Read the model definition and answer for the solid it produces. Units are mm, in the model's axes. Face numbers are marked on the shaded views. A direction names the side the tool comes from. Give positions to 0.01 mm unless a question says otherwise; leave off trailing zeros. Order: outer loops, then holes, each group sorted by start corner. A loop starts at its lowest first (then second) coordinate and runs counter-clockwise, first axis right, second up. Notation, with made-up numbers: (88, 43) -> (128, 43) arc R13 ccw to (128, 64) -> close; hole circle Ø3 at (9, 1). An arc over 180 degrees is marked (long way). One line per item, written item: value. Start each with the question number.
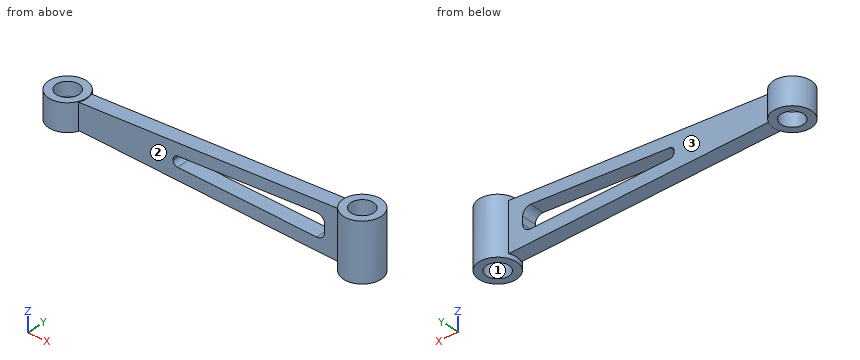
from build123d import *

# Parameters (mm, degrees)
SKETCH1_R           = 7.5
BOSS_EXTRUDE1_DEPTH = 9
SKETCH2_R           = 7.5
BOSS_EXTRUDE2_DEPTH = 19
BOSS_EXTRUDE3_DEPTH = 5
SKETCH4_R           = 12.5
BOSS_EXTRUDE4_DEPTH = 9
SKETCH6_R           = 12.5
BOSS_EXTRUDE5_DEPTH = 19
SKETCH7_R           = 7.5
CUT_EXTRUDE1_DEPTH  = 19
CUT_EXTRUDE2_DEPTH  = 19


with BuildPart() as part:
    # Sketch1 → Boss-Extrude1 (new body, symmetric)
    with BuildSketch(Plane.XY):
        Circle(SKETCH1_R)
    extrude(amount=BOSS_EXTRUDE1_DEPTH, both=True)



with BuildPart() as body_2:
    # Sketch2 → Boss-Extrude2 (new body, symmetric)
    with BuildSketch(Plane.XY):
        with Locations((194.56, 0)):
            Circle(SKETCH2_R)
    extrude(amount=BOSS_EXTRUDE2_DEPTH, both=True)


with BuildPart() as body_3:
    # Sketch3 → Boss-Extrude3 (new body, symmetric)
    with BuildSketch(Plane(origin=(0, 0, 0), x_dir=(1, 0, 0), z_dir=(0, 1, 0))):
        Polygon((7.5, 8.362970839), (187.06, 16.2), (187.06, -16.20477539), (7.5, -8.362286729), align=None)
    extrude(amount=BOSS_EXTRUDE3_DEPTH, both=True)


with BuildPart() as part_1:
    add(part.part)

    add(body_3.part)  # Boss-Extrude4 merges body 3
    # Sketch4 → Boss-Extrude4 (add, symmetric)
    with BuildSketch(Plane.XY):
        Circle(SKETCH4_R)
    extrude(amount=BOSS_EXTRUDE4_DEPTH, both=True)


    add(body_2.part)  # Boss-Extrude5 merges body 2
    # Sketch6 → Boss-Extrude5 (add, symmetric)
    with BuildSketch(Plane.XY):
        with Locations((194.56, 0)):
            Circle(SKETCH6_R)
    extrude(amount=BOSS_EXTRUDE5_DEPTH, both=True)

    # Sketch7 → Cut-Extrude1 (cut, symmetric)
    with BuildSketch(Plane.XY):
        Circle(SKETCH7_R)
        with Locations((194.56, 0)):
            Circle(SKETCH7_R)
    extrude(amount=CUT_EXTRUDE1_DEPTH, both=True, mode=Mode.SUBTRACT)

    # Sketch8 → Cut-Extrude2 (cut, symmetric)
    with BuildSketch(Plane(origin=(0, 5, 0), x_dir=(1, 0, 0), z_dir=(0, 1, 0))):
        with BuildLine():
            Line((76.769384169, 3.36885549), (168.688973616, 7.067498603))
            ThreePointArc((168.688973616, 7.067498603), (172.353731231, 5.677448491), (173.89, 2.071541398))
            Line((173.89, 2.071541398), (173.89, -2.721863896))
            ThreePointArc((173.89, -2.721863896), (172.341389234, -6.33958588), (168.654835057, -7.716330579))
            Line((168.654835057, -7.716330579), (76.748901034, -3.388930862))
            ThreePointArc((76.748901034, -3.388930862), (74.719366809, -2.463084392), (73.89, -0.392250852))
            Line((73.89, -0.392250852), (73.89, 0.371281167))
            ThreePointArc((73.89, 0.371281167), (74.726455744, 2.449519905), (76.769384169, 3.36885549))
        make_face()
    extrude(amount=CUT_EXTRUDE2_DEPTH, both=True, mode=Mode.SUBTRACT)


solid = part_1.part
Item 1: Find section B-B on y = 0. Write down the section's boundary in (x, z), then the cut area to 3 significant figures.
Item 2: Flat-ended cylindrical pins translate along their axes: pin 1 (6 mm diameter, centred on x = 175, y = -4, fed in from +Z); pin 2 (4 mm diameter, centred on x = 163.5, y = 1.5, fed in from +Z); pin 3 (9 mm diameter, centred on x = 194.56, y = 0, fed in from +Z); pin 4 (8 mm diameter, centred on y = -5, z = -7.5, fed in from +X). Find the tip coordinate at first contact, or state that the pin passes through.
Item 3: Find the intervals of material crossed by line 1 (Y direction, x = 194.56, z = -4); line 2 (X direction, y = 3.5, z = 8); line 3 (X direction, y = 10, z = -3), in increasing order. Write a range as from..to.
Item 4: Find section D-D on x = 194.56. Write down the section's boundary in (y, z), then the cut area to 3 significant figures.
Item 5: A tool of negligible diameter and unlimited length cuts with its end or side. For the marked faces 1, 2 and 3, from which of +Z, -Z, +X, -X, +Y, -Y can it reach the whole face along a straight path? Write none if from no direction.
Item 6: Find section A-A on x = 0. Write down the section's boundary in (y, z), then the cut area to 3 significant figures.
Item 7: Find section C-C on z = 12. Write down the section's boundary in (x, y).
Checks:
1. outline: (-12.5, -9) -> (-7.5, -9) -> (-7.5, 9) -> (-12.5, 9) -> close; (7.5, -9) -> (12.5, -9) -> (12.5, -8.58) -> (182.06, -15.98) -> (182.06, -19) -> (187.06, -19) -> (187.06, 19) -> (182.06, 19) -> (182.06, 15.99) -> (12.5, 8.58) -> (12.5, 9) -> (7.5, 9) -> close; (202.06, -19) -> (207.06, -19) -> (207.06, 19) -> (202.06, 19) -> close; hole (73.89, -0.37) arc R3 ccw to (76.77, -3.37) -> (168.69, -7.07) arc R5 ccw to (173.89, -2.07) -> (173.89, 2.72) arc R5 ccw to (168.65, 7.72) -> (76.75, 3.39) arc R3 ccw to (73.89, 0.39) -> close
1. area: 3,650 mm2
2. pin 1: z = 15.81
2. pin 2: z = 15.26
2. pin 3: through
2. pin 4: x = 207.02
3. line 1: -12.5..-7.5, 7.5..12.5
3. line 2: -12..-6.63, 6.63..187.93, 201.19..206.56
3. line 3: -7.5..7.5, 187.06..202.06
4. outline: (-12.5, -19) -> (-7.5, -19) -> (-7.5, 19) -> (-12.5, 19) -> close; (7.5, -19) -> (12.5, -19) -> (12.5, 19) -> (7.5, 19) -> close
4. area: 380 mm2
5. face 1: +Z, -Z
5. face 2: +Z, -Z, -Y
5. face 3: +Z, -Z, +Y
6. outline: (-12.5, -9) -> (-7.5, -9) -> (-7.5, 9) -> (-12.5, 9) -> close; (7.5, -9) -> (12.5, -9) -> (12.5, 9) -> (7.5, 9) -> close
6. area: 180 mm2
7. outline: (90.79, -5) -> (183.1, -5) arc R12.5 ccw (long way) to (183.1, 5) -> (90.79, 5) -> close; hole circle Ø15 at (194.56, 0)
